Can you work these out from the model? Positions are in its coordinate system, mm. A direction names the side the tool comes from. Round coordinates to 2 decimals unless told otherwise and drop trailing zeros. Order: outer loops, then holes, each group sorted by start corner. A loop starts at its lowest first (then second) coordinate and runs counter-clockwise, first axis right, second up. Notation, with made-up numbers: M 36,29.25 L 55,29.25 A22 cw 55,59.25 Z; hole C 89.5,40.5 d5. An arc over 180 degrees is marked long. Answer as a JSON object with one key per item and string values. Group by question number.
from build123d import *

# Parameters (mm, degrees)
PAD_DEPTH     = 43
SKETCH001_W   = 85
SKETCH001_H   = 50
SKETCH001_W_2 = 8
SKETCH001_H_2 = 15
PAD001_DEPTH  = 3
SKETCH002_R   = 2.5
PAD002_DEPTH  = 48


with BuildPart() as part:
    # Sketch → Pad (new body)
    with BuildSketch(Plane.XZ):
        with BuildLine():
            Line((-43, 28), (43, 28))
            ThreePointArc((45.5, 25.5), (44.767767, 27.267767), (43, 28))
            Line((45.5, 25.5), (45.5, -25.5))
            ThreePointArc((43, -28), (44.767767, -27.267767), (45.5, -25.5))
            Line((43, -28), (-43, -28))
            ThreePointArc((-45.5, -25.5), (-44.767767, -27.267767), (-43, -28))
            Line((-45.5, -25.5), (-45.5, 25.5))
            ThreePointArc((-43, 28), (-44.767767, 27.267767), (-45.5, 25.5))
        make_face()
        with BuildLine():
            Line((-40.55051, 25), (40.55051, 25))
            ThreePointArc((40.55051, 25), (41.232233, 23.732233), (42.5, 23.05051))
            Line((42.5, 23.05051), (42.5, -23.05051))
            ThreePointArc((42.5, -23.05051), (41.232233, -23.732233), (40.55051, -25))
            Line((40.55051, -25), (-40.55051, -25))
            ThreePointArc((-40.55051, -25), (-41.232233, -23.732233), (-42.5, -23.05051))
            Line((-42.5, -23.05051), (-42.5, 23.05051))
            ThreePointArc((-42.5, 23.05051), (-41.232233, 23.732233), (-40.55051, 25))
        make_face(mode=Mode.SUBTRACT)
    extrude(amount=PAD_DEPTH)

    # Sketch001 → Pad001 (join)
    with BuildSketch(Plane.XZ):
        Rectangle(SKETCH001_W, SKETCH001_H)
        with Locations((-28.5, 0)):
            Rectangle(SKETCH001_W_2, SKETCH001_H_2, mode=Mode.SUBTRACT)
    extrude(amount=PAD001_DEPTH)

    # Sketch002 → Pad002 (join)
    with BuildSketch(Plane.XZ):
        with Locations((-43, 25.5)):
            Circle(SKETCH002_R)
        with Locations((43, 25.5)):
            Circle(SKETCH002_R)
        with Locations((43, -25.5)):
            Circle(SKETCH002_R)
        with Locations((-43, -25.5)):
            Circle(SKETCH002_R)
    extrude(amount=PAD002_DEPTH)


solid = part.part
Item 1: On a 3-axis mill with a long thin cutter (end or side, diameter ignored), from which of +Z, -Z, +X, -X, +Y, -Y can I reach the whole of each face in a straight line? I mean faces 1 (the face through (42.5, -23, 0)), 2 (the face through (-45.5, -21, 0)), 3 (the face through (-24.5, -1, 0)). Say none if no direction works.
Item 2: Suppose I cut it at B-B, the plane x = 37. Write out the boundary of the cut face in (y, z).
Item 3: I'm going to push flat-ended pins straight in: pin 1 Ø0.9 at (x, z) = (-44.5, 4) entering from -Y; pin 2 Ø10 at (x, z) = (35, 18.5) entering from +Y. Where does each tip first touch, or does it pass through?
Item 4: Suppose I cut it at C-C, the plane z = -10.5. Write out the boundary of the cut face in (x, y), and give its area (3 significant figures).
Item 5: Suppose I cut it at A-A, the plane y = -21.5. Write out the boundary of the cut face in (x, z).
Item 6: I need wall thicknesses on line 1 (Z direction, x = 14, y = -26.5); line 2 (X direction, y = -5.5, z = 6); line 3 (Z direction, x = 41, y = -16). Which ranges of each line are inside material? Lowest first, please.
Item 7: If we mould it in two halves opening along Z, with no side actions, what happens to faces 4 (the face through (-29, -1, 7.5)), 5 (the face through (43, -48, -25)), 6 (the face through (-1, -21, 28))? For each: +Z half, -Z half, draft (parallel to the pull), parting line (faces both ways), or undercut.
Computed:
{
 "1": {"face 1": "-Y", "face 2": "+Z, -Z, -X, +Y, -Y", "face 3": "+Y, -Y"},
 "2": {"outline": "M -43,-28 L 0,-28 L 0,28 L -43,28 L -43,25 L -3,25 L -3,-25 L -43,-25 Z"},
 "3": {"pin 1": "stops at y = -43", "pin 2": "stops at y = 0"},
 "4": {"outline": "M -45.5,-43 L -42.5,-43 L -42.5,-3 L 42.5,-3 L 42.5,-43 L 45.5,-43 L 45.5,0 L -45.5,0 Z", "area": "513 mm^2"},
 "5": {"outline": "M -45.5,-25.5 A2.5 ccw -43,-28 L 43,-28 A2.5 ccw 45.5,-25.5 L 45.5,25.5 A2.5 ccw 43,28 L -43,28 A2.5 ccw -45.5,25.5 Z; hole M -42.5,-23.05 A2.5 cw -40.55,-25 L 40.55,-25 A2.5 cw 42.5,-23.05 L 42.5,23.05 A2.5 cw 40.55,25 L -40.55,25 A2.5 cw -42.5,23.05 Z"},
 "6": {"line 1": "z = -28 to -25, 25 to 28", "line 2": "x = -45.5 to -42.5, 42.5 to 45.5", "line 3": "z = -28 to -24, 24 to 28"},
 "7": {"face 4": "undercut", "face 5": "draft", "face 6": "+Z half"}
}
